```python
from build123d import *

# Parameters (mm, degrees)
ESQUISSE1_R                   = 3.5
BOSS_EXTRU_1_DEPTH            = 44
ESQUISSE2_R                   = 2
BOSS_EXTRU_2_DEPTH            = 5
ESQUISSE3_R                   = 1.5
BOSS_EXTRU_3_DEPTH            = 0.5
ESQUISSE4_R                   = 2
BOSS_EXTRU_4_DEPTH            = 1.5
CHANFREIN1_SIZE               = 0.5
CHANFREIN2_SIZE               = 0.5
DIAM_TRE_DU_PER_AGE_2_0_2_3_D = 2


with BuildPart() as part:
    # Esquisse1 → Boss.-Extru.1 (new body)
    with BuildSketch(Plane.XY):
        Circle(ESQUISSE1_R)
    extrude(amount=BOSS_EXTRU_1_DEPTH)

    # Esquisse2 → Boss.-Extru.2 (add)
    with BuildSketch(Plane.XY.offset(44)):
        Circle(ESQUISSE2_R)
    extrude(amount=BOSS_EXTRU_2_DEPTH)

    # Esquisse3 → Boss.-Extru.3 (add)
    with BuildSketch(Plane.XY.offset(49)):
        Circle(ESQUISSE3_R)
    extrude(amount=BOSS_EXTRU_3_DEPTH)

    # Esquisse4 → Boss.-Extru.4 (add)
    with BuildSketch(Plane.XY.offset(49.5)):
        Circle(ESQUISSE4_R)
    extrude(amount=BOSS_EXTRU_4_DEPTH)

    # Chanfrein1
    chanfrein1_edges = [part.edges().sort_by_distance(p)[0] for p in [
        (-2, 0, 51),
    ]]
    chamfer(chanfrein1_edges, length=CHANFREIN1_SIZE)

    # Chanfrein2
    chanfrein2_edges = [part.edges().sort_by_distance(p)[0] for p in [
        (-3.5, 0, 0),
    ]]
    chamfer(chanfrein2_edges, length=CHANFREIN2_SIZE)

    # Diamètre du perçage Ø2.0 (2)3 (through all)
    with Locations(Plane(origin=(0, 3.5, 5.615), x_dir=(1, 0, 0), z_dir=(0, 1, 0))):
        with Locations((0, 0)):
            Hole(DIAM_TRE_DU_PER_AGE_2_0_2_3_D / 2)


solid = part.part
```
The listing builds one solid part. Answer for the finished solid, in the listing's coordinates (mm). A direction names the side the tool comes from. Coordinates: 2 decimals unless noted, no trailing zeros. Write each loop counter-clockwise with the first axis right and the second up, starting at its lowest first coordinate (ties: lowest second). Pieces come first, ordered by that corner, then holes. Notation, with made-up numbers: (51, 73.5) -> (74, 73.5) arc R20 cw to (74, 86.5) -> close; hole circle Ø8 at (-26.5, 30). An arc over 180 degrees is marked (long way). Write each question's results on one line, items separated by ' | '. Start each with the question number.
1) A cutting plane is placed at B-B (y = 0). Determine the outline of the cut face in (x, z) (3 decimals).
2) A cutting plane is placed at C-C (z = 39). Determine the outline of the cut face in (x, y), then the cut area to 3 significant figures.
3) For a pull along Z with two mould halves and no side action, classify faces 3 (the cylindrical face through (-1.5, 0.07, 49.25)), 4 (the cylindrical face through (0.22, -0.05, 6.59)), 5 (the flat face through (2, -2, 44)), 6 (the cylindrical face through (0, -2, 50)) as +Z half, -Z half, draft (parallel to the pull), parting line (faces both ways), or undercut.
4) A cutting plane is placed at A-A (x = 0). Determine the outline of the cut face in (y, z) (3 decimals), then the cut area to 3 significant figures.
5) Straight lines are drawn through the part: probe 1 along Z at (x, y) = (0, 1.25) (3 decimals); probe 2 along Z at (x, y) = (0, 1.75) (3 decimals); probe 3 along Z at (x, y) = (2.25, 2). For each, find the intervals that lie inside material, in ascending order.
6) Flat-ended cylindrical pins translate along their axes: pin 1 Ø1.5 at (x, z) = (2, 33) entering from -Y; pin 2 Ø3 at (x, z) = (2, 36) entering from +Y; pin 3 Ø3 at (y, z) = (2.5, 12.5) entering from -X. Find the tip coordinate at first contact, or state that the pin passes through.
7) A tool of negligible diameter and unlimited length cuts with its end or side. For faces 1 (the flat face through (0, 0, 51)), 2 (the cylindrical face through (0, -2, 46)), from which of +Z, -Z, +X, -X, +Y, -Y can it reach the whole face along a straight path? Write none if from no direction.
Values follow:
1) outline: (-3.5, 0.5) -> (-3, 0) -> (3, 0) -> (3.5, 0.5) -> (3.5, 44) -> (2, 44) -> (2, 49) -> (1.5, 49) -> (1.5, 49.5) -> (2, 49.5) -> (2, 50.5) -> (1.5, 51) -> (-1.5, 51) -> (-2, 50.5) -> (-2, 49.5) -> (-1.5, 49.5) -> (-1.5, 49) -> (-2, 49) -> (-2, 44) -> (-3.5, 44) -> close; hole circle Ø2 at (0, 5.615)
2) outline: circle Ø7 at (0, 0) | area: 38.5 mm²
3) face 3: undercut | face 4: undercut | face 5: +Z half | face 6: draft
4) outline: (-3.5, 0.5) -> (-3, 0) -> (3, 0) -> (3.5, 0.5) -> (3.5, 4.615) -> (-3.5, 4.615) -> close; (-3.5, 6.615) -> (3.5, 6.615) -> (3.5, 44) -> (2, 44) -> (2, 49) -> (1.5, 49) -> (1.5, 49.5) -> (2, 49.5) -> (2, 50.5) -> (1.5, 51) -> (-1.5, 51) -> (-2, 50.5) -> (-2, 49.5) -> (-1.5, 49.5) -> (-1.5, 49) -> (-2, 49) -> (-2, 44) -> (-3.5, 44) -> close | area: 321 mm²
5) probe 1: 0 to 4.615, 6.615 to 51 | probe 2: 0 to 4.615, 6.615 to 49, 49.5 to 50.75 | probe 3: 0.01 to 44
6) pin 1: y = -3.27 | pin 2: y = 3.46 | pin 3: x = -3.35
7) face 1: +Z, +X, -X, +Y, -Y | face 2: +Z
